from build123d import *

# Parameters (mm, degrees)
SKETCH_1_W      = 3
SKETCH_1_H      = 10
SKETCH_1_W_2    = 10
SKETCH_1_H_2    = 3
SKETCH_1_R      = 1.5
EXTRUDE_1_DEPTH = 1.5
SKETCH_1_3_W    = 3
SKETCH_1_3_H    = 10
EXTRUDE_2_DEPTH = 2.5
EXTRUDE_START   = 1.5
SKETCH_1_4_W    = 3
SKETCH_1_4_H    = 3
EXTRUDE_3_DEPTH = 1


with BuildPart() as part:
    # Эскиз1 → Бобышка-Вытянуть1 (new body)
    with BuildSketch(Plane(origin=(0, 0, 0), x_dir=(1, 0, 0), z_dir=(0, 1, 0))):
        with Locations((-5, 0)):
            Rectangle(SKETCH_1_W, SKETCH_1_H)
        with Locations((1.5, 0)):
            Rectangle(SKETCH_1_W_2, SKETCH_1_H)
        with Locations((4, -2.5)):
            Rectangle(SKETCH_1_W, SKETCH_1_H_2, mode=Mode.SUBTRACT)
        with Locations((4, 2.5)):
            Circle(SKETCH_1_R, mode=Mode.SUBTRACT)
        with Locations((4, -2.5)):
            Rectangle(SKETCH_1_W, SKETCH_1_H_2)
    extrude(amount=EXTRUDE_1_DEPTH)

    # Эскиз1<3> → Бобышка-Вытянуть2 (add)
    with BuildSketch(Plane(origin=(0, 0, 0), x_dir=(1, 0, 0), z_dir=(0, 1, 0))):
        with Locations((-5, 0)):
            Rectangle(SKETCH_1_3_W, SKETCH_1_3_H)
    extrude(amount=-EXTRUDE_2_DEPTH)

    # Эскиз1<4> → Бобышка-Вытянуть3 (add)
    with BuildSketch(Plane(origin=(0, 0, 0), x_dir=(1, 0, 0), z_dir=(0, 1, 0)).offset(EXTRUDE_START)):
        with Locations((4, -2.5)):
            Rectangle(SKETCH_1_4_W, SKETCH_1_4_H)
    extrude(amount=EXTRUDE_3_DEPTH)


solid = part.part
Model file for the job. Use its own axes, mm. A direction names the side the tool comes from. Coordinates: 2 decimals unless noted, no trailing zeros. Loops run counter-clockwise (first coordinate to the right, second up) from the corner with the lowest first, then second, coordinate; pieces in that order, holes last. Notation, with made-up numbers: (-32, 31.25) -> (-25, 31.25) arc R25 cw to (-25, 65.25) -> close; hole circle Ø3 at (23.25, 75). An arc over 180 degrees is marked (long way). Use one line per item in the form item = value. Start each with the question number.
(1) Cut at D-D on z = 2.75. Give the cut face in (x, y), and give its area (3 significant figures).
(2) Tool access for faces 5 (the flat face through (4, 2, 1)), 6 (the flat face through (4, 2, 4)), 7 (the flat face through (5.5, 2, 3)), 8 (the flat face through (2.5, 2, 3)), 9 (the flat face through (-3.5, -1, 0)): list every direction of +Z, -Z, +X, -X, +Y, -Y with a clear straight run to the whole face (end or side of a thin tool).
(3) Pull direction Z, two halves, no side cores. Call faces 1 (the cylindrical face through (5.386, 0.74, -1.925)), 2 (the flat face through (-1.5, 0.4, 5)), 3 (the flat face through (-1.5, 0.4, -5)), 4 (the flat face through (6.5, 1, 0)): pulls with the +Z half, pulls with the -Z half, needs draft (parallel to the pull), parting line crosses it, or undercut.
(4) Cut at C-C on y = 0.9. Give the cut face in (x, z).
(5) Cut at A-A on x = 4. Give the cut face in (y, z).
(6) Flat gauge pins, fed straight in: pin 1 (5 mm diameter, centred on x = 2.5, z = 2, fed in from -Y); pin 2 (0.5 mm diameter, centred on x = 4, y = 2, fed in from -Z); pin 3 (0.8 mm diameter, centred on y = 2, z = 2, fed in from -X). Where does each tip first touch, or does it go through?
(7) Probe probe 1 along Z at (x, y) = (4, 1); probe 2 along X at (y, z) = (1.1, -2.5); probe 3 along Y at (x, z) = (-4.5, 3.5). List the from-to ranges inside material, lowest first. Write a range as from..to.
(8) Cut at B-B on z = -2.5. Give the cut face in (x, y), and give its area (3 significant figures).
Values:
q1.outline = (-6.5, -2.5) -> (-3.5, -2.5) -> (-3.5, 0) -> (6.5, 0) -> (6.5, 1.5) -> (5.5, 1.5) -> (5.5, 2.5) -> (2.5, 2.5) -> (2.5, 1.5) -> (-6.5, 1.5) -> close
q1.area = 30.0 mm2
q2.face_5 = -Z, +X, -X, +Y
q2.face_6 = +Z, +X, -X, +Y
q2.face_7 = +Z, -Z, +X, +Y
q2.face_8 = +Z, -Z, -X, +Y
q2.face_9 = +Z, -Z, +X, -Y
q3.face_1 = undercut
q3.face_2 = pulls with the +Z half
q3.face_3 = pulls with the -Z half
q3.face_4 = needs draft
q4.outline = (-6.5, -5) -> (6.5, -5) -> (6.5, 5) -> (-6.5, 5) -> close; hole circle Ø3 at (4, -2.5)
q5.outline = (0, -5) -> (1.5, -5) -> (1.5, -4) -> (0, -4) -> close; (0, -1) -> (1.5, -1) -> (1.5, 1) -> (2.5, 1) -> (2.5, 4) -> (1.5, 4) -> (1.5, 5) -> (0, 5) -> close
q6.pin_1 = 0
q6.pin_2 = 1
q6.pin_3 = 2.5
q7.probe_1 = -5..-4, -1..5
q7.probe_2 = -6.5..2.5, 5.5..6.5
q7.probe_3 = -2.5..1.5
q8.outline = (-6.5, -2.5) -> (-3.5, -2.5) -> (-3.5, 0) -> (2.5, 0) -> (2.5, 1.5) -> (-6.5, 1.5) -> close; (5.5, 0) -> (6.5, 0) -> (6.5, 1.5) -> (5.5, 1.5) -> close
q8.area = 22.5 mm2
